Input: part model. Units: mm. Frame: model coordinates. Face numbers are marked on the shaded views. Give positions to 0.01 mm unless a question says otherwise; leave off trailing zeros. Loops run counter-clockwise (first coordinate to the right, second up) from the corner with the lowest first, then second, coordinate; pieces in that order, holes last. Notation, with made-up numbers: M 23,25.5 L 49,25.5 A24 cw 49,55.5 Z; hole C -7,32 d6. An arc over 180 degrees is marked long. Answer as a JSON object with one key per item and string values. Group by question number.
1) Section query B-B on z = 12. Return loops of the section in (x, y), plus the area to 3 significant figures.
2) Ray query, L1, parallel to X at y = 1, z = 2.75; L2, parallel to Y at x = -0.75, z = -2; L3, parallel to Z at x = 1, y = 6.75 (3 decimals). Return the intervals inside material, ascending.
3) Section query A-A on z = 5. Return loops of the section in (x, y).
4) Draft query along Y for the marked faces 1, 2 and 3. Return one class per face: +Y half, -Y half, draft (parallel to the pull), parting line (faces both ways), or undercut.
5) First-contact query: P1, Ø1, axis at x = 4.5, y = 2, coming from the -Z side; P2, Ø1.5, axis at x = -5, y = 1, coming from the +Z side; P3, Ø2, axis at y = -3.5, z = 10, coming from the +X side. Flat tips, straight axial feed; report the tip coordinate or a pass-through.
from build123d import *

# Parameters (mm, degrees)
F3_R = 0.762


# Not quite as in the source:
# - a feature names something its author has since deleted; it is built from what else it names


with BuildPart() as f2:
    # F0 (on Front) → F2 (revolve)
    with BuildSketch(Plane.XZ):
        with BuildLine():
            Line((3.8862, 1.0368246978), (3.8862, 11.7048246978))
            ThreePointArc((3.8862, 11.7048246978), (2.8543707216, 12.645076528), (1.6046219265, 13.2670677765))
            Line((1.6046219265, 13.2670677765), (0, 12.9230134189))
            Line((0, 12.9230134189), (0, -0.635))
            add(Edge.make_bspline(
                [(6.0325, -3.175), (4.927107133, -1.9561804365), (4.0449600812, -1.3553717475), (1.9983640724, -0.7115763161), (0.9248232606, -0.5421136513), (0, -0.635)],
                knots=[0, 0, 0, 0, 0.3804425123, 0.6767184943, 1, 1, 1, 1], degree=3))
            Line((6.0325, -3.175), (11.1125, -3.175))
            add(Edge.make_bspline(
                [(5.207, 1.0368246978), (5.7984997261, 0.975644811), (6.74291899, 0.5105425669), (9.2830121982, -0.5417734643), (10.4753485066, -2.2706511595), (11.1125, -3.175)],
                knots=[0, 0, 0, 0, 0.2725407329, 0.6170084006, 1, 1, 1, 1], degree=3))
            Line((5.207, 1.0368246978), (3.8862, 1.0368246978))
        make_face()
    revolve(axis=Axis((0, 0, 1.4091059566), (0, 0, -1)))

    # F3
    f3_edges = [f2.edges().sort_by_distance(p)[0] for p in [
        (-1.604622, 0, 13.267068),
        (-6.0325, 0, -3.175),
        (-11.1125, 0, -3.175),
    ]]
    fillet(f3_edges, radius=F3_R)


solid = f2.part
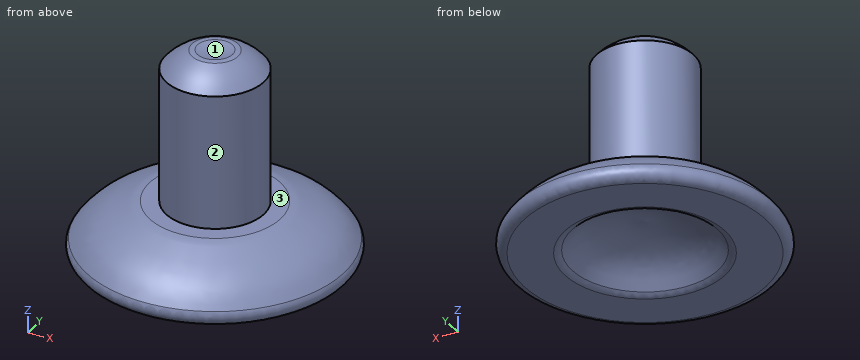
Output:
{
 "1": {"outline": "C 0,0 d7.24", "area": "41.2 mm^2"},
 "2": {"L1": "x = -3.76 to 3.76", "L2": "y = -10.23 to -4.79, 4.79 to 10.23", "L3": "z = -3.175 to 0.498"},
 "3": {"outline": "C 0,0 d7.77"},
 "4": {"face 1": "undercut", "face 2": "parting line", "face 3": "draft"},
 "5": {"P1": "stops at z = -2.53", "P2": "stops at z = 1.04", "P3": "stops at x = 2.98"}
}
